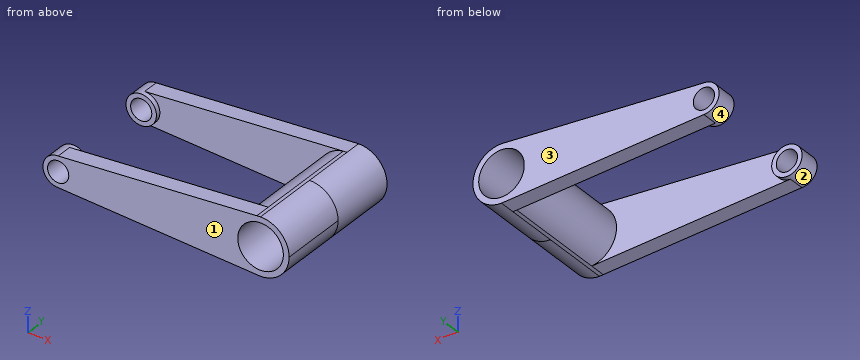
from build123d import *

# Parameters (mm, degrees)
CROQUIS11_R             = 9.320716026
CROQUIS11_R_2           = 6.498904475
SALIENTE_EXTRUIR7_DEPTH = 13
SALIENTE_EXTRUIR8_DEPTH = 10
CROQUIS11_17_R          = 13.974913408
SALIENTE_EXTRUIR9_DEPTH = 42.662603
SIMETR_A3_START         = 75.325206553
SIMETR_A3_OUTLINE_R     = 6.498904475
SIMETR_A3_OUTLINE_R_2   = 13.974913408
SIMETR_A3_DEPTH         = 10
SIMETR_A3_START_2       = 42.662603276
SIMETR_A3_2_OUTLINE_R   = 13.974913408
SIMETR_A3_2_DEPTH       = 32.662603277
SIMETR_A3_START_3       = 72.325206553
SIMETR_A3_3_OUTLINE_R   = 9.320716026
SIMETR_A3_3_OUTLINE_R_2 = 6.498904475
SIMETR_A3_3_DEPTH       = 3


# Read off the part's stored shape, not the designer's step: Simetría3
with BuildPart() as part:
    # Croquis11 → Saliente-Extruir7 (new body)
    with BuildSketch(Plane(origin=(0, 0, 0), x_dir=(1, 0, 0), z_dir=(0, 1, 0))):
        with Locations(Location((5.950503047, 0, 0), (0, 0, 90))):
            Circle(CROQUIS11_R)
        with Locations(Location((5.950503047, 0, 0), (0, 0, 90))):
            Circle(CROQUIS11_R_2, mode=Mode.SUBTRACT)
    extrude(amount=SALIENTE_EXTRUIR7_DEPTH)

    # Croquis11<13> → Saliente-Extruir8 (add)
    with BuildSketch(Plane(origin=(0, 0, 0), x_dir=(1, 0, 0), z_dir=(0, 1, 0))):
        with BuildLine():
            Line((112.450503047, 0), (15.271219073, 0))
            ThreePointArc((15.271219073, 0), (12.541244554, -6.590741507), (5.950503047, -9.320716026))
            Line((5.950503047, -9.320716026), (127.651835642, -17.348375375))
            ThreePointArc((127.651835642, -17.348375375), (116.788499408, -11.533068118), (112.450503047, 0))
        make_face()
        with BuildLine():
            ThreePointArc((5.950503047, 9.320716026), (12.541244554, 6.590741507), (15.271219073, 0))
            Line((15.271219073, 0), (112.450503047, 0))
            ThreePointArc((112.450503047, 0), (116.788499408, 11.533068118), (127.651835642, 17.348375375))
            Line((127.651835642, 17.348375375), (5.950503047, 9.320716026))
        make_face()
    extrude(amount=SALIENTE_EXTRUIR8_DEPTH)

    # Croquis11<17> → Saliente-Extruir9 (add)
    with BuildSketch(Plane(origin=(0, 0, 0), x_dir=(1, 0, 0), z_dir=(0, 1, 0))):
        with BuildLine():
            ThreePointArc((127.651835642, 17.348375375), (112.450503047, 0), (127.651835642, -17.348375375))
            Line((127.651835642, -17.348375375), (129.950503047, -17.5))
            ThreePointArc((129.950503047, -17.5), (142.324871718, -12.374368671), (147.450503047, 0))
            ThreePointArc((147.450503047, 0), (142.324871718, 12.374368671), (129.950503047, 17.5))
            Line((129.950503047, 17.5), (127.651835642, 17.348375375))
        make_face()
        with Locations(Location((129.950503047, 0, 0), (0, 0, 270))):
            Circle(CROQUIS11_17_R, mode=Mode.SUBTRACT)
    extrude(amount=SALIENTE_EXTRUIR9_DEPTH)



with BuildPart() as body_2:
    # Simetría3 outline → Simetría3 (new body)
    with BuildSketch(Plane(origin=(0, 0, 0), x_dir=(1, 0, 0), z_dir=(0, 1, 0)).offset(SIMETR_A3_START)):
        with BuildLine():
            ThreePointArc((5.950503047, 9.320716026), (-3.370212979, 0), (5.950503047, -9.320716026))
            Line((5.950503047, -9.320716026), (129.950503047, -17.5))
            ThreePointArc((129.950503047, -17.5), (147.450503047, 0), (129.950503047, 17.5))
            Line((129.950503047, 17.5), (5.950503047, 9.320716026))
        make_face()
        with Locations((5.950503047, 0)):
            Circle(SIMETR_A3_OUTLINE_R, mode=Mode.SUBTRACT)
        with Locations((129.950503047, 0)):
            Circle(SIMETR_A3_OUTLINE_R_2, mode=Mode.SUBTRACT)
    extrude(amount=SIMETR_A3_DEPTH)


with BuildPart() as part_1:
    add(part.part)

    add(body_2.part)  # Simetr_a3 2 merges body 2
    # Simetr_a3 2 outline → Simetr_a3 2 (add)
    with BuildSketch(Plane(origin=(0, 0, 0), x_dir=(1, 0, 0), z_dir=(0, 1, 0)).offset(SIMETR_A3_START_2)):
        with BuildLine():
            Line((129.950503047, 17.5), (127.651835642, 17.348375375))
            ThreePointArc((127.651835642, 17.348375375), (112.450503047, 0), (127.651835642, -17.348375375))
            Line((127.651835642, -17.348375375), (129.950503047, -17.5))
            ThreePointArc((129.950503047, -17.5), (147.450503047, 0), (129.950503047, 17.5))
        make_face()
        with Locations((129.950503047, 0)):
            Circle(SIMETR_A3_2_OUTLINE_R, mode=Mode.SUBTRACT)
    extrude(amount=SIMETR_A3_2_DEPTH)

    # Simetr_a3 3 outline → Simetr_a3 3 (add)
    with BuildSketch(Plane(origin=(0, 0, 0), x_dir=(1, 0, 0), z_dir=(0, 1, 0)).offset(SIMETR_A3_START_3)):
        with Locations((5.950503047, 0)):
            Circle(SIMETR_A3_3_OUTLINE_R)
        with Locations((5.950503047, 0)):
            Circle(SIMETR_A3_3_OUTLINE_R_2, mode=Mode.SUBTRACT)
    extrude(amount=SIMETR_A3_3_DEPTH)


solid = part_1.part
Read the model definition and answer for the solid it produces. Units are mm, in the model's axes. Face numbers are marked on the shaded views. A direction names the side the tool comes from. Give positions to 0.01 mm unless a question says otherwise; leave off trailing zeros. Write each loop counter-clockwise with the first axis right and the second up, starting at its lowest first coordinate (ties: lowest second). Pieces come first, ordered by that corner, then holes. Notation, with made-up numbers: (-19.75, -9.5) - (26.25, -9.5) arc R22 cw to (26.25, 10.5) - close; hole circle Ø7 at (-12.75, 64). An arc over 180 degrees is marked (long way). Answer in a Markdown table with one row per item. Add a question column.
Item 1: Find the intervals of material crossed by L1, parallel to X at y = 78, z = 0; L2, parallel to Y at x = 78.5, z = -12.5; L3, parallel to X at y = 14, z = 0.5, in increasing order.
Item 2: A tool of negligible diameter and unlimited length cuts with its end or side. For the marked faces 3 and 4, from which of +Z, -Z, +X, -X, +Y, -Y can it reach the whole face along a straight path? Write none if from no direction.
Item 3: Determine the mould class of the marked faces 1 and 2 for opening direction X: pulls with the +X half, pulls with the -X half, needs draft (parallel to the pull), parting line crosses it, or undercut.
Item 4: Section D-D, the plane x = 134 is taken. Write down the section's boundary in (y, z).
Item 5: Section C-C, the plane z = -3 is taken. Write down the section's boundary in (x, y).
Item 6: Section B-B, the plane x = 42 is taken. Write down the section's boundary in (y, z).
Item 7: Section A-A, the plane y = 39.5 is taken. Write down the section's boundary in (x, z).
Item 8: Flat-ended cylindrical pins translate along their axes: P1, Ø4, axis at y = 41.5, z = 2.5, coming from the +X side; P2, Ø8, axis at x = 5.95, z = 0, coming from the -Y side; P3, Ø8, axis at y = 65, z = 3.5, coming from the -X side. Find the tip coordinate at first contact, or state that the pin passes through.
Recorded:
| question | item | result |
|---|---|---|
| 1 | L1 | x = -3.37 to -0.55, 12.45 to 115.98, 143.93 to 147.45 |
| 1 | L2 | y = 0 to 10, 75.33 to 85.33 |
| 1 | L3 | x = 112.46 to 115.98, 143.92 to 147.44 |
| 2 | face 3 | +Z, -Z, +X, -X, +Y |
| 2 | face 4 | none |
| 3 | face 1 | needs draft |
| 3 | face 2 | undercut |
| 4 | outline | (0, -17.03) - (85.33, -17.03) - (85.33, -13.38) - (0, -13.38) - close; (0, 13.38) - (85.33, 13.38) - (85.33, 17.03) - (0, 17.03) - close |
| 5 | outline | (-2.87, 0) - (0.19, 0) - (0.19, 13) - (-2.87, 13) - close; (-2.87, 72.33) - (0.19, 72.33) - (0.19, 85.33) - (-2.87, 85.33) - close; (11.72, 0) - (116.3, 0) - (116.3, 85.33) - (11.72, 85.33) - (11.72, 72.33) - (14.78, 72.33) - (14.78, 75.33) - (112.71, 75.33) - (112.71, 10) - (14.78, 10) - (14.78, 13) - (11.72, 13) - close; (143.6, 0) - (147.19, 0) - (147.19, 85.33) - (143.6, 85.33) - close |
| 6 | outline | (0, -11.7) - (10, -11.7) - (10, 11.7) - (0, 11.7) - close; (75.33, -11.7) - (85.33, -11.7) - (85.33, 11.7) - (75.33, 11.7) - close |
| 7 | outline | (127.65, -17.35) - (129.95, -17.5) arc R17.5 ccw to (129.95, 17.5) - (127.65, 17.35) arc R17.5 ccw to start; hole circle Ø27.95 at (129.95, 0) |
| 8 | P1 | stops at x = 147.44 |
| 8 | P2 | passes through |
| 8 | P3 | stops at x = 112.45 |
